Read the model definition and answer for the solid it produces. Units are mm, in the model's axes. Face numbers are marked on the shaded views. A direction names the side the tool comes from. Give positions to 0.01 mm unless a question says otherwise; leave off trailing zeros. Write each loop counter-clockwise with the first axis right and the second up, starting at its lowest first coordinate (ties: lowest second). Pieces come first, ordered by that corner, then holes. Notation, with made-up numbers: (19, -29) - (52, -29) arc R14 cw to (52, -4) - close; hole circle Ø3 at (71, 66). An arc over 180 degrees is marked (long way). Answer as a JSON object with one key per item and string values. Group by question number.
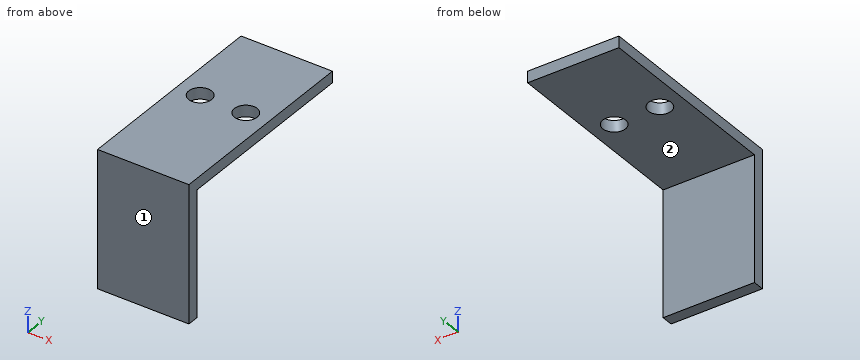
```python
from build123d import *

# Parameters (mm, degrees)
BOSS_EXTRUDE1_DEPTH = 25.4
SKETCH2_R           = 3.175
CUT_EXTRUDE1_DEPTH  = 72.631264997


with BuildPart() as part:
    # Sketch1 → Boss-Extrude1 (new body)
    with BuildSketch(Plane(origin=(0, 0, 0), x_dir=(0, 0, -1), z_dir=(1, 0, 0))):
        Polygon((38.1, 0), (38.1, 3.175), (3.175, 3.175), (3.175, 57.15), (0, 57.15), (0, 0), align=None)
    extrude(amount=BOSS_EXTRUDE1_DEPTH)

    # Sketch2 → Cut-Extrude1 (cut, through all)
    with BuildSketch(Plane(origin=(0, 0, -3.175), x_dir=(-1, 0, 0), z_dir=(0, 0, -1))):
        with Locations((-19.05, 31.75)):
            Circle(SKETCH2_R)
        with Locations((-6.35, 31.75)):
            Circle(SKETCH2_R)
    extrude(amount=-CUT_EXTRUDE1_DEPTH, mode=Mode.SUBTRACT)


solid = part.part
```
1) Find section D-D, the plane x = 21.5. Write down the section's boundary in (y, z) (3 decimals).
2) Find section B-B, the plane x = 6.35. Write down the section's boundary in (y, z) (3 decimals), and give its area (3 significant figures).
3) Find section A-A, the plane y = 31.75. Write down the section's boundary in (x, z) (3 decimals), and give its area (3 significant figures).
4) Find section C-C, the plane z = -11.5. Write down the section's boundary in (x, y) (3 decimals), and give its area (3 significant figures).
5) Flat-ended cylindrical pins translate along their axes: pin 1 Ø12.5 at (x, y) = (13, 41.5) entering from -Z (3 decimals); pin 2 Ø4 at (x, y) = (19.05, 31.75) entering from -Z; pin 3 Ø7.5 at (x, z) = (9.5, -17.5) entering from +Y (3 decimals). Find the tip coordinate at first contact, or state that the pin passes through.
6) Which of the six approach directions +Z, -Z, +X, -X, +Y, -Y give full straight-line access (tool end or side, diameter ignored) to the marked faces 1 and 2?
7) Find the intervals of material crossed by line 1 (Y direction, x = 6.35, z = -2.1) (3 decimals); line 2 (X direction, y = 31, z = -2); line 3 (Y direction, x = 6.75, z = -12) (3 decimals), in increasing order. Write a range as [from, to].
Values follow:
{
 "1": {"outline": "(0, -38.1) - (3.175, -38.1) - (3.175, -3.175) - (29.731, -3.175) - (29.731, 0) - (0, 0) - close; (33.769, -3.175) - (57.15, -3.175) - (57.15, 0) - (33.769, 0) - close"},
 "2": {"outline": "(0, -38.1) - (3.175, -38.1) - (3.175, -3.175) - (28.575, -3.175) - (28.575, 0) - (0, 0) - close; (34.925, -3.175) - (57.15, -3.175) - (57.15, 0) - (34.925, 0) - close", "area": "272 mm2"},
 "3": {"outline": "(0, -3.175) - (3.175, -3.175) - (3.175, 0) - (0, 0) - close; (9.525, -3.175) - (15.875, -3.175) - (15.875, 0) - (9.525, 0) - close; (22.225, -3.175) - (25.4, -3.175) - (25.4, 0) - (22.225, 0) - close", "area": "40.3 mm2"},
 "4": {"outline": "(0, 0) - (25.4, 0) - (25.4, 3.175) - (0, 3.175) - close", "area": "80.6 mm2"},
 "5": {"pin 1": "stops at z = -3.175", "pin 2": "passes through", "pin 3": "stops at y = 3.175"},
 "6": {"face 1": "+Z, -Z, +X, -X, -Y", "face 2": "-Z, +X, -X, +Y"},
 "7": {"line 1": "y = [0, 28.575], [34.925, 57.15]", "line 2": "x = [0, 3.26], [9.44, 15.96], [22.14, 25.4]", "line 3": "y = [0, 3.175]"}
}
